from build123d import *

# Parameters (mm, degrees)
F0_W     = 130.175
F0_H     = 60.325
F1_DEPTH = 44.45
F3_W     = 34.9023286253
F3_H     = 60.4157168418
F4_DEPTH = 44.45
F5_DEPTH = 25.4
F7_DEPTH = 60.325
F8_W     = 44.45
F8_H     = 60.325
F9_DEPTH = 34.925


with BuildPart() as f1:
    # F0 (on Front) → F1 (new body)
    with BuildSketch(Plane.XZ):
        with Locations((1.020533964, -6.2578915411)):
            Rectangle(F0_W, F0_H)
    extrude(amount=F1_DEPTH)

    # F3 (on face) → F4 (cut)
    with BuildSketch(Plane.XZ.offset(44.45)):
        with Locations((48.6795557663, -6.1232140288)):
            Rectangle(F3_W, F3_H)
    extrude(amount=-F4_DEPTH, mode=Mode.SUBTRACT)

    # F5 (cut): a face of the model
    f5_faces = [f1.faces().sort_by_distance(p)[0] for p in [
        (48.6682127088, -22.225, -36.3310724497),
    ]]
    extrude(f5_faces, amount=-F5_DEPTH, mode=Mode.SUBTRACT)

    # F6 (on face) → F7 (cut)
    with BuildSketch(Plane.YZ.offset(31.2283914536)):
        Polygon((-44.45, 23.9046084589), (-44.45, -23.7203915411), (-16.9536934298, 23.9046084589), align=None)
    extrude(amount=-F7_DEPTH, mode=Mode.SUBTRACT)

    # F8 (on face) → F9 (join)
    with BuildSketch(Plane.YZ.offset(31.2283914536)):
        with Locations((-22.225, -6.2578915411)):
            Rectangle(F8_W, F8_H)
    extrude(amount=F9_DEPTH)


solid = f1.part
Design review of the part built by this model. Coordinates are the model's own, in mm. A direction names the side the tool comes from. Coordinates: 2 decimals unless noted, no trailing zeros. Order: outer loops, then holes, each group sorted by start corner. A loop starts at its lowest first (then second) coordinate and runs counter-clockwise, first axis right, second up. Notation, with made-up numbers: M 27.5,-14.75 L 46.5,-14.75 A16 ccw 46.5,14.25 Z; hole C 39,58.5 d6. An arc over 180 degrees is marked long. Use a Markdown table: item, result.
(1) For faces 1 (the flat face through (-29.097, -34, 6)), 2 (the flat face through (0, -44.45, -27)), list the 3-axis set-ups (+Z, -Z, +X, -X, +Y, -Y) from which the entire face can be reached by the end or side of a thin tool; tool diameter is ignored.
Worked answers:
| item | result |
|---|---|
| face 1 | +Z, -Y |
| face 2 | +Z, -Z, +X, -X, -Y |
(2) Wall thickness on probe 1 along X at (y, z) = (-29, 6.5); probe 2 along Z at (x, y) = (2, -19); probe 3 along Z at (x, y) = (23, -36.5): over which ranges is each line inside the solid? List them lowest first.
Worked answers:
| item | result |
|---|---|
| probe 1 | x = -64.07 to -29.1, 31.23 to 66.15 |
| probe 2 | z = -36.42 to 20.36 |
| probe 3 | z = -36.42 to -9.95 |
(3) Draft analysis for pull direction X (two halves, no side actions). For faces 3 (the flat face through (66.153, -23, -6)), 4 (the flat face through (0, 0, -7)), 5 (the flat face through (1.488, -30.894, -0.241)), state which applies: released by +X, released by -X, zero draft, split by the parting line, or undercut.
Worked answers:
| item | result |
|---|---|
| face 3 | released by +X |
| face 4 | zero draft |
| face 5 | undercut |
(4) Add section B-B (x = -10.5). Give the boundary of the cut face in (y, z).
Worked answers:
| item | result |
|---|---|
| outline | M -44.45,-36.42 L 0,-36.42 L 0,23.9 L -16.95,23.9 L -44.45,-23.72 Z |
(5) Add section A-A (z = -2). Give the boundary of the cut face in (x, y).
Worked answers:
| item | result |
|---|---|
| outline | M -64.07,-44.45 L -29.1,-44.45 L -29.1,-31.91 L 31.23,-31.91 L 31.23,-44.45 L 66.15,-44.45 L 66.15,0 L -64.07,0 Z |
(6) Add section C-C (y = -24). Give the boundary of the cut face in (x, z), then the cut area to 3 significant figures.
Worked answers:
| item | result |
|---|---|
| outline | M -64.07,-36.42 L 66.15,-36.42 L 66.15,23.9 L 31.23,23.9 L 31.23,11.7 L -29.1,11.7 L -29.1,23.9 L -64.07,23.9 Z |
| area | 7,120 mm2 |
(7) For P1, Ø5, axis at x = -24.5, y = -18.5, coming from the +Z side, flat-tipped, find the tip position at first contact; note if it passes through.
Worked answers:
| item | result |
|---|---|
| P1 | stops at z = 23.9 |
